Read the model definition and answer for the solid it produces. Units are mm, in the model's axes. Face numbers are marked on the shaded views. Round coordinates to 2 decimals unless told otherwise and drop trailing zeros. Order: outer loops, then holes, each group sorted by start corner. A loop starts at its lowest first (then second) coordinate and runs counter-clockwise, first axis right, second up. Notation, with made-up numbers: (81.5, -16) -> (132.5, -16) arc R15 cw to (132.5, 9) -> close; hole circle Ø11 at (52, -31.75). An arc over 180 degrees is marked (long way). Answer as a JSON object with one key per item and string values. Group by question number.
Item 1: Section B-B, the plane y = 1.25 is taken. Write down the section's boundary in (x, z).
Item 2: Section D-D, the plane y = -1.75 is taken. Write down the section's boundary in (x, z), plus the area to 3 significant figures.
Item 3: Section A-A, the plane x = -10.5 is taken. Write down the section's boundary in (y, z), plus the area to 3 significant figures.
Item 4: The mould has two halves that part along Y. Classify the marked faces 1, 2 and 3: pulls with the +Y half, pulls with the -Y half, needs draft (parallel to the pull), parting line crosses it, or undercut.
Item 5: Consider probe 1 along Y at (x, z) = (-6, 1.15); probe 2 along X at (y, z) = (4.5, 2.15); probe 3 along X at (y, z) = (1.25, 1.7). Determine where each line is inside the solid, lowest interval first. Write a range as from..to.
Item 6: Section C-C, the plane z = 2.9 is taken. Write down the section's boundary in (x, y), plus the area to 3 significant figures.
Item 7: Given P1, Ø7, axis at x = -7.2, y = 3.5, coming from the -Z side; P2, Ø1, axis at y = 3, z = 2, coming from the +X side, each flat-ended and moving along its own axis, determine where each tip first touches the part or whether it passes through.
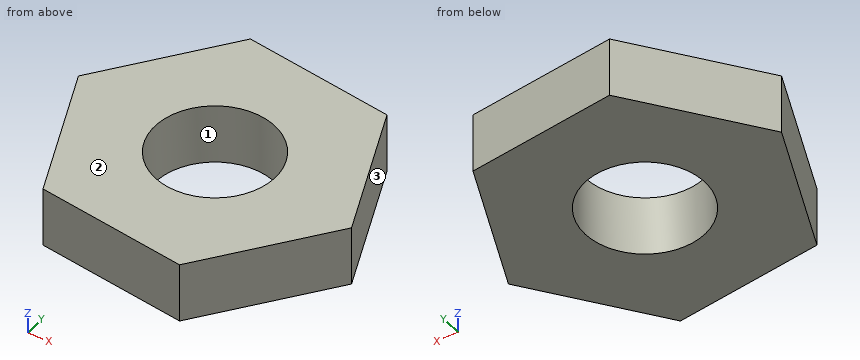
from build123d import *

# Parameters (mm, degrees)
BOSS_EXTRUDE1_DEPTH = 4
SKETCH2_R           = 4
CUT_EXTRUDE1_DEPTH  = 4


with BuildPart() as part:
    # Sketch1 → Boss-Extrude1 (new body)
    with BuildSketch(Plane.XY):
        Polygon((2.730304444, 2.302220599), (-1.198694049, 11.498033279), (-11.127000685, 12.693327112), (-17.126308828, 4.692808266), (-13.197310334, -4.503004414), (-3.269003699, -5.698298248), align=None)
    extrude(amount=BOSS_EXTRUDE1_DEPTH)

    # Sketch2 → Cut-Extrude1 (cut)
    with BuildSketch(Plane.XY.offset(4)):
        with Locations((-7.198002192, 3.497514432)):
            Circle(SKETCH2_R)
    extrude(amount=-CUT_EXTRUDE1_DEPTH, mode=Mode.SUBTRACT)


solid = part.part
Values found:
{
 "1": {"outline": "(-15.66, 0) -> (-10.51, 0) -> (-10.51, 4) -> (-15.66, 4) -> close; (-3.89, 0) -> (1.94, 0) -> (1.94, 4) -> (-3.89, 4) -> close"},
 "2": {"outline": "(-14.37, 0) -> (-0.31, 0) -> (-0.31, 4) -> (-14.37, 4) -> close", "area": "56.3 mm2"},
 "3": {"outline": "(-4.83, 0) -> (1.24, 0) -> (1.24, 4) -> (-4.83, 4) -> close; (5.76, 0) -> (12.62, 0) -> (12.62, 4) -> (5.76, 4) -> close", "area": "51.7 mm2"},
 "4": {"face 1": "undercut", "face 2": "needs draft", "face 3": "pulls with the +Y half"},
 "5": {"probe 1": "-5.37..-0.32, 7.31..12.08", "probe 2": "-17.04..-11.07, -3.33..1.79", "probe 3": "-15.66..-10.51, -3.89..1.94"},
 "6": {"outline": "(-17.13, 4.69) -> (-13.2, -4.5) -> (-3.27, -5.7) -> (2.73, 2.3) -> (-1.2, 11.5) -> (-11.13, 12.69) -> close; hole circle Ø8 at (-7.2, 3.5)", "area": "210 mm2"},
 "7": {"P1": "through", "P2": "x = 2.65"}
}
